Geometry: final body of the model. Coordinates: model frame, mm. A direction names the side the tool comes from. Round coordinates to 2 decimals unless told otherwise and drop trailing zeros. Loops run counter-clockwise (first coordinate to the right, second up) from the corner with the lowest first, then second, coordinate; pieces in that order, holes last. Notation, with made-up numbers: (-5.75, 85) - (26.25, 85) arc R28 ccw to (26.25, 109) - close; hole circle Ø4 at (-31, 6). An arc over 180 degrees is marked (long way). Write item = value, one per line. Start each with the question number.
Item 1: Section D-D (x = 12). Return loops of the section in (y, z).
Item 2: Draft query along Y for faces 1 (the flat face through (-50.444, 2.362, 1.972)), 2 (the cylindrical face through (-1.956, 5.022, 1.972)), 3 (the flat face through (-29.538, 17.417, 1.972)), 4 (the flat face through (-3, 3, 0)). Return one class per face: pulls with the +Y half, pulls with the -Y half, needs draft (parallel to the pull), parting line crosses it, or undercut.
Item 3: Section A-A (z = 2.3). Return loops of the section in (x, y), plus the area to 3 significant figures.
Item 4: Access query for faces 5 (the flat face through (5, 48, 2)), 6 (the flat face through (-9, 48, 2)), 7 (the flat face through (-4, 17, 2)), 8 (the flat face through (-23.253, 26.487, 1.972)). Directions: +Z, -Z, +X, -X, +Y, -Y. A direction counts if a zero-diameter tool reaches every point of the face in a straight line with its end or side. Return the directions, or none.
Item 5: Section C-C (y = 45). Return loops of the section in (x, z), plus the area to 3 significant figures.
Item 6: Line query: line 1 (X direction, y = 50.5, z = 0.45); line 2 (X direction, y = 27, z = 0.25); line 3 (X direction, y = 23, z = 1). Output: solid intervals per line, ascending. Write a range as from..to.
Item 7: Section B-B (x = -2). Return loops of the section in (y, z), plus the area to 3 significant figures.
Item 8: First-contact query: pin 1 (1 mm diameter, centred on y = 34, z = 2, fed in from +X); pin 2 (2 mm diameter, centred on y = 46.5, z = 2.5, fed in from +X). Flat tips, straight axial feed; report the tip coordinate or a pass-through.
from build123d import *

# Parameters (mm, degrees)
F1_DEPTH = 4


with BuildPart() as f1:
    # F0 (on Top) → F1 (new body)
    with BuildSketch(Plane.XY):
        Polygon((-24.640209, 27.888809), (-21.827112, 25.045134), (-37.467321, 9.5731), (-40.280418, 12.416774), (-60.897057, -7.978181), (56.897057, -7.978181), (36.280418, 12.416774), (33.467321, 9.5731), (17.827112, 25.045134), (20.640209, 27.888809), (5, 43.360843), (5, 53.360843), (-9, 53.360843), (-9, 43.360843), align=None)
        with BuildLine():
            Line((0, 27.021819), (0, 7.021819))
            ThreePointArc((0, 7.021819), (-2, 5.021819), (-4, 7.021819))
            Line((-4, 7.021819), (-4, 27.021819))
            ThreePointArc((-4, 27.021819), (-2, 29.021819), (0, 27.021819))
        make_face(mode=Mode.SUBTRACT)
    extrude(amount=F1_DEPTH)


solid = f1.part
Taken from the geometry:
q1.outline = (-7.98, 0) - (36.44, 0) - (36.44, 4) - (-7.98, 4) - close
q2.face_1 = pulls with the +Y half
q2.face_2 = undercut
q2.face_3 = undercut
q2.face_4 = needs draft
q3.outline = (-60.9, -7.98) - (56.9, -7.98) - (36.28, 12.42) - (33.47, 9.57) - (17.83, 25.05) - (20.64, 27.89) - (5, 43.36) - (5, 53.36) - (-9, 53.36) - (-9, 43.36) - (-24.64, 27.89) - (-21.83, 25.05) - (-37.47, 9.57) - (-40.28, 12.42) - close; hole (-4, 7.02) arc R2 ccw to (0, 7.02) - (0, 27.02) arc R2 ccw to (-4, 27.02) - close
q3.area = 3,250 mm^2
q4.face_5 = +Z, -Z, +X, +Y
q4.face_6 = +Z, -Z, -X, +Y
q4.face_7 = +Z, -Z
q4.face_8 = +Z, -Z, -X
q5.outline = (-9, 0) - (5, 0) - (5, 4) - (-9, 4) - close
q5.area = 56.0 mm^2
q6.line_1 = -9..5
q6.line_2 = -23.76..-4, 0..19.76
q6.line_3 = -23.89..-4, 0..19.89
q7.outline = (-7.98, 0) - (5.02, 0) - (5.02, 4) - (-7.98, 4) - close; (29.02, 0) - (53.36, 0) - (53.36, 4) - (29.02, 4) - close
q7.area = 149 mm^2
q8.pin_1 = 14.97
q8.pin_2 = 5
